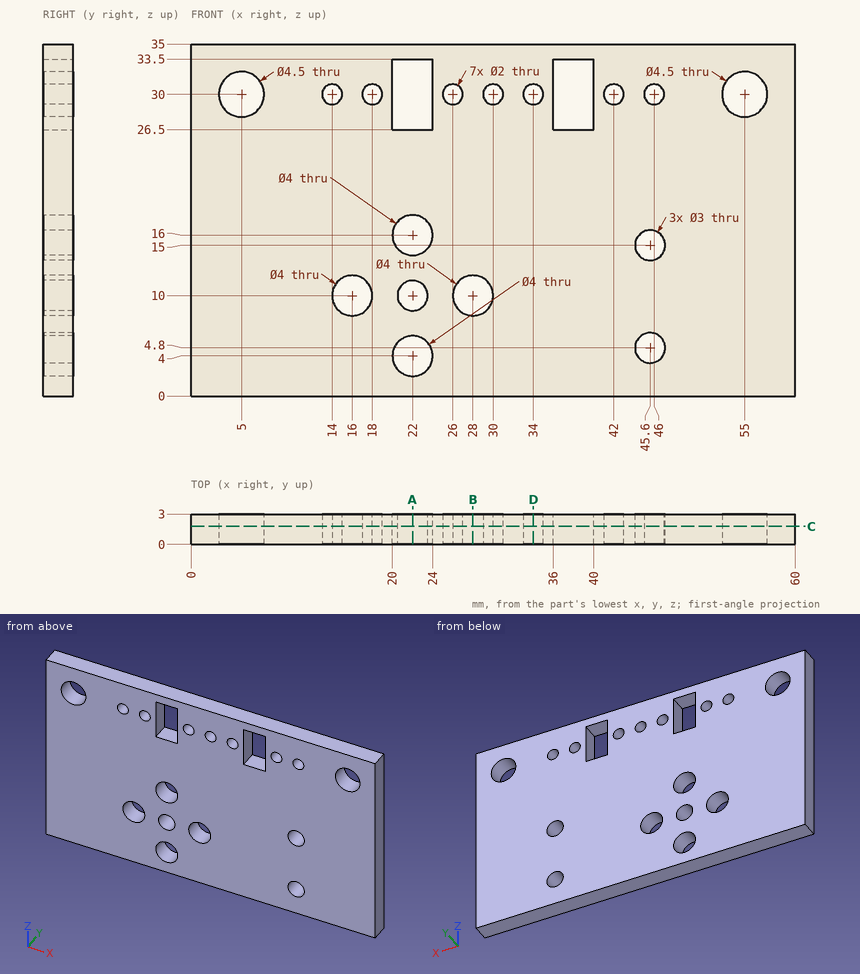
Here's the drawing with two shaded views (mm, measured from the low corner). I have some questions. Round coordinates to 2 decimals unless told otherwise and drop trailing zeros. Write each loop counter-clockwise with the first axis right and the second up, starting at its lowest first coordinate (ties: lowest second). Pieces come first, ordered by that corner, then holes.
(1) Suppose I cut it at C-C on y = 1.8. State how many separate pieces and enclosed holes the cut face has, and give its area (3 significant figures).
Findings below:
separate pieces: 1
enclosed holes: 18
area: 1,920 mm2
(2) For pin 1 (6 mm diameter, centred on x = 5, z = 30, fed in from +Y); pin 2 (3 mm diameter, centred on x = 28, z = 10, fed in from +Y), each with a flat end and sliding along its axis, tell me the tip position at first contact or that it passes through.
Findings below:
pin 1: stops at y = 3
pin 2: passes through
(3) Suppose I cut it at B-B on x = 28. Write out the boundary of the cut face in (y, z).
Findings below:
outline: (0, 0) - (3, 0) - (3, 8) - (0, 8) - close; (0, 12) - (3, 12) - (3, 35) - (0, 35) - close
(4) Suppose I cut it at A-A on x = 22. Write out the boundary of the cut face in (y, z), and give its area (3 significant figures).
Findings below:
outline: (0, 0) - (3, 0) - (3, 2) - (0, 2) - close; (0, 6) - (3, 6) - (3, 8.5) - (0, 8.5) - close; (0, 11.5) - (3, 11.5) - (3, 14) - (0, 14) - close; (0, 18) - (3, 18) - (3, 26.5) - (0, 26.5) - close; (0, 33.5) - (3, 33.5) - (3, 35) - (0, 35) - close
area: 51.0 mm2
(5) Suppose I cut it at D-D on x = 34. Write out the boundary of the cut face in (y, z), and give its area (3 significant figures).
Findings below:
outline: (0, 0) - (3, 0) - (3, 29) - (0, 29) - close; (0, 31) - (3, 31) - (3, 35) - (0, 35) - close
area: 99.0 mm2
(6) If I drill on probe 1 along Z at (x, y) = (39, 1.5); probe 2 along X at (y, z) = (1.15, 33); probe 3 along Z at (x, y) = (46, 0.95), over which ranges is the centre line in solid material (lowest first)?
Findings below:
probe 1: z = 0 to 26.5, 33.5 to 35
probe 2: x = 0 to 20, 24 to 36, 40 to 60
probe 3: z = 0 to 3.35, 6.25 to 13.55, 16.45 to 29, 31 to 35
